Design review of the part built by this model. Coordinates are the model's own, in mm. A direction names the side the tool comes from. Give positions to 0.01 mm unless a question says otherwise; leave off trailing zeros. Write each loop counter-clockwise with the first axis right and the second up, starting at its lowest first coordinate (ties: lowest second). Pieces come first, ordered by that corner, then holes. Notation, with made-up numbers: (-22, 27) -> (-17, 27) arc R17 cw to (-17, 45) -> close; hole circle Ø2 at (60, -26). An arc over 180 degrees is marked (long way). Write each question's results on one line, items separated by ' | '. Start each with the question number.
(1) Take a section at D-D (z = -9.3). State the section outline as (x, y) points.
(2) Take a section at A-A (x = 41.5). State the section outline as (y, z) points.
(3) Take a section at B-B (x = 19.5). State the section outline as (y, z) points.
(4) To check wall thickness, follow probe 1 along X at (y, z) = (1.2, -4.5); probe 2 along Z at (x, y) = (41.5, 1.05); probe 3 along X at (y, z) = (0.4, -0.5). State the ranges of each line that lie inside material, in increasing order.
(5) For faces 1 (the face through (31, 1, -12.27)), 2 (the face through (30, 1, 12.73)), 3 (the face through (10.5, 1, 0)), list the 3-axis set-ups (+Z, -Z, +X, -X, +Y, -Y) from which the entire face can be reached by the end or side of a thin tool; tool diameter is ignored.
(6) Clearance check with a flat-ended pin moving along its axis: pin 1 (0.5 mm diameter, centred on y = 1, z = 16.5, fed in from +X). State where the tip first meets the part, or that it passes through.
(7) Take a section at C-C (z = 0.5). State the section outline as (x, y) points.
(8) Mouldability with a two-part tool opening along Z and no side actions: class faces 4 (the face through (16, 1, 17)), 5 (the face through (14, 1, -19.77)), 6 (the face through (17, 1, 5.8)) as released by +Z, released by -Z, zero draft, split by the parting line, or undercut.
from build123d import *

# Parameters (mm, degrees)
BOSS_EXTRUDE1_DEPTH = 1.6
CUT_EXTRUDE1_DEPTH  = 0.56
SKETCH3_W           = 13
SKETCH3_H           = 11.6
CUT_EXTRUDE2_DEPTH  = 2
SKETCH4_R           = 0.75
CUT_EXTRUDE3_DEPTH  = 2


with BuildPart() as part:
    # Sketch1 → Boss-Extrude1 (new body)
    with BuildSketch(Plane(origin=(0, 0, 0), x_dir=(1, 0, 0), z_dir=(0, 1, 0))):
        Polygon((0, 6), (0, -6), (11, -20.23), (16, -20.23), (16, -12.73), (45, -12.73), (45, 12.27), (16, 12.27), (16, 19.77), (11, 19.77), align=None)
    extrude(amount=BOSS_EXTRUDE1_DEPTH)

    # Sketch2 → Cut-Extrude1 (cut)
    with BuildSketch(Plane(origin=(0, 1.6, 0), x_dir=(1, 0, 0), z_dir=(0, 1, 0))):
        Polygon((0, -6), (9.5, -18.289545455), (9.5, 17.892272727), (0, 6), (1.5, 6), (1.5, -6), align=None)
    extrude(amount=-CUT_EXTRUDE1_DEPTH, mode=Mode.SUBTRACT)

    # Sketch3 → Cut-Extrude2 (cut)
    with BuildSketch(Plane(origin=(0, 1.6, 0), x_dir=(1, 0, 0), z_dir=(0, 1, 0))):
        with Locations((17, 0)):
            Rectangle(SKETCH3_W, SKETCH3_H)
    extrude(amount=-CUT_EXTRUDE2_DEPTH, mode=Mode.SUBTRACT)

    # Sketch4 → Cut-Extrude3 (cut)
    with BuildSketch(Plane(origin=(0, 1.6, 0), x_dir=(1, 0, 0), z_dir=(0, 1, 0))):
        with Locations(Location((13.5, 16.27, 0), (0, 0, 270))):
            Circle(SKETCH4_R)
        with Locations(Location((13.5, 9.3, 0), (0, 0, 270))):
            Circle(SKETCH4_R)
        with Locations(Location((41.5, 9.3, 0), (0, 0, 270))):
            Circle(SKETCH4_R)
        with Locations(Location((41.5, -9.3, 0), (0, 0, 270))):
            Circle(SKETCH4_R)
        with Locations(Location((13.5, -9.3, 0), (0, 0, 270))):
            Circle(SKETCH4_R)
        with Locations(Location((13.5, -16.73, 0), (0, 0, 270))):
            Circle(SKETCH4_R)
    extrude(amount=-CUT_EXTRUDE3_DEPTH, mode=Mode.SUBTRACT)


solid = part.part
Report:
1) outline: (2.64, 0) -> (12.75, 0) -> (12.75, 1.6) -> (9.5, 1.6) -> (9.5, 1.04) -> (2.64, 1.04) -> close; (14.25, 0) -> (40.75, 0) -> (40.75, 1.6) -> (14.25, 1.6) -> close; (42.25, 0) -> (45, 0) -> (45, 1.6) -> (42.25, 1.6) -> close
2) outline: (0, -12.27) -> (1.6, -12.27) -> (1.6, -10.05) -> (0, -10.05) -> close; (0, -8.55) -> (1.6, -8.55) -> (1.6, 8.55) -> (0, 8.55) -> close; (0, 10.05) -> (1.6, 10.05) -> (1.6, 12.73) -> (0, 12.73) -> close
3) outline: (0, -12.27) -> (1.6, -12.27) -> (1.6, -5.8) -> (0, -5.8) -> close; (0, 5.8) -> (1.6, 5.8) -> (1.6, 12.73) -> (0, 12.73) -> close
4) probe 1: 0 to 1.5, 9.5 to 10.5, 23.5 to 45 | probe 2: -12.27 to -10.05, -8.55 to 8.55, 10.05 to 12.73 | probe 3: 0 to 10.5, 23.5 to 45
5) face 1: -Z, +X, +Y, -Y | face 2: +Z, +X, +Y, -Y | face 3: +Y, -Y
6) pin 1: x = 16
7) outline: (0, 0) -> (10.5, 0) -> (10.5, 1.6) -> (9.5, 1.6) -> (9.5, 1.04) -> (1.5, 1.04) -> (1.5, 1.6) -> (0, 1.6) -> close; (23.5, 0) -> (45, 0) -> (45, 1.6) -> (23.5, 1.6) -> close
8) face 4: zero draft | face 5: released by -Z | face 6: undercut
